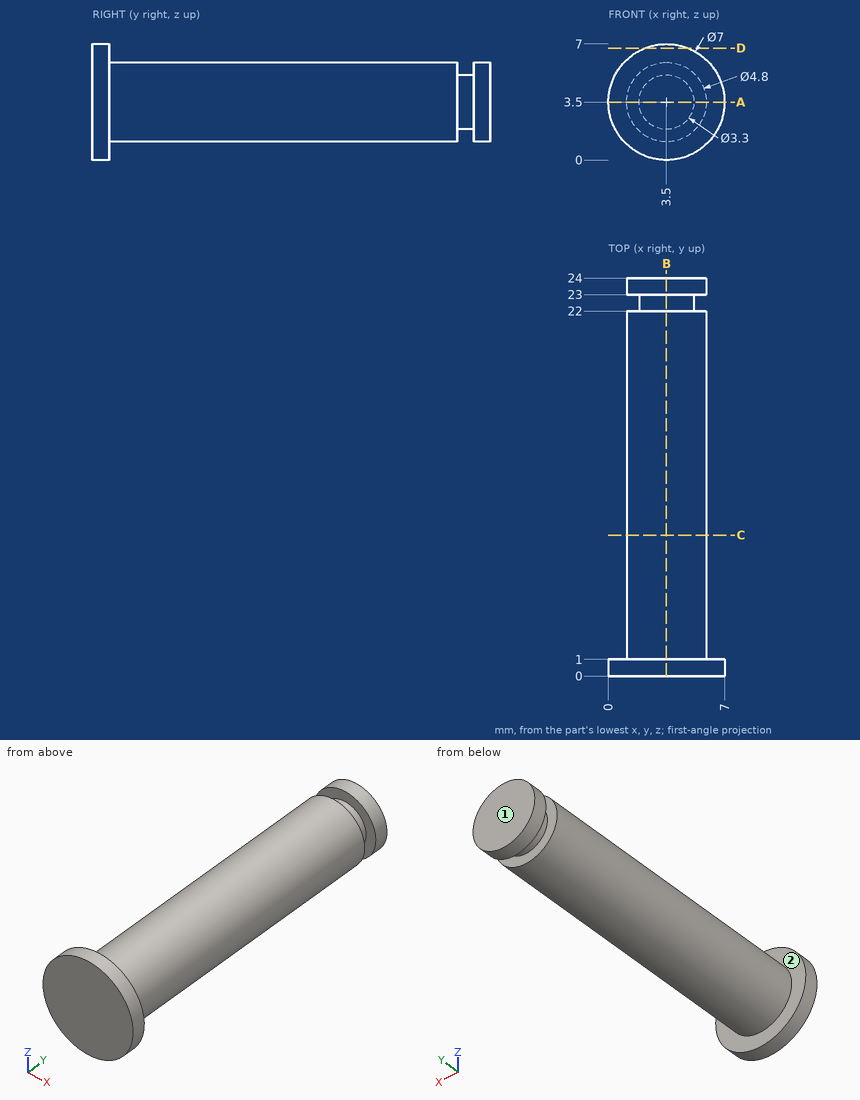
Here's the drawing with two shaded views (mm, measured from the low corner). I have some questions. A direction names the side the tool comes from. Give positions to 0.01 mm unless a question says otherwise; leave off trailing zeros. Loops run counter-clockwise (first coordinate to the right, second up) from the corner with the lowest first, then second, coordinate; pieces in that order, holes last. Notation, with made-up numbers: M -6,36.25 L 25,36.25 A15 cw 25,61.25 Z; hole C 56.5,15 d2. An arc over 180 degrees is marked long. Use one line per item in the form item = value. Start each with the question number.
(1) On a 3-axis mill with a long thin cutter (end or side, diameter ignored), from which of +Z, -Z, +X, -X, +Y, -Y can I reach the whole of each face in a straight line? I mean the marked faces 1 and 2. Say none if no direction works.
(2) I'm going to push flat-ended pins straight in: P1, Ø3, axis at y = 11.5, z = 5.5, coming from the +X side; P2, Ø4, axis at x = 3, y = 7.5, coming from the +Z side; P3, Ø2, axis at y = 19.5, z = 1, coming from the -X side. Where does each tip first touch, or does it pass through?
(3) I want a section at C-C, the plane y = 8.5. Write out the boundary of the cut face in (x, z), and give its area (3 significant figures).
(4) I want a section at B-B, the plane x = 3.5. Write out the boundary of the cut face in (y, z).
(5) I want a section at D-D, the plane z = 6.75. Write out the boundary of the cut face in (x, y), and give its area (3 significant figures).
(6) I want a section at A-A, the plane z = 3.5. Write out the boundary of the cut face in (x, y).
(7) Please list where these lines run through material, in increasing order: line 1 (Y direction, x = 2, z = 4.25); line 2 (Y direction, x = 1.75, z = 1.5); line 3 (X direction, y = 13, z = 2.75).
Worked out:
q1.face_1 = +Z, -Z, +X, -X, +Y
q1.face_2 = +Y
q2.P1 = 5.85
q2.P2 = 5.9
q2.P3 = 1.63
q3.outline = C 3.5,3.5 d4.8
q3.area = 18.1 mm²
q4.outline = M 0,0 L 1,0 L 1,1.1 L 22,1.1 L 22,1.85 L 23,1.85 L 23,1.1 L 24,1.1 L 24,5.9 L 23,5.9 L 23,5.15 L 22,5.15 L 22,5.9 L 1,5.9 L 1,7 L 0,7 Z
q5.outline = M 2.2,0 L 4.8,0 L 4.8,1 L 2.2,1 Z
q5.area = 2.60 mm²
q6.outline = M 0,0 L 7,0 L 7,1 L 5.9,1 L 5.9,22 L 5.15,22 L 5.15,23 L 5.9,23 L 5.9,24 L 1.1,24 L 1.1,23 L 1.85,23 L 1.85,22 L 1.1,22 L 1.1,1 L 0,1 Z
q7.line_1 = 0 to 22, 23 to 24
q7.line_2 = 0 to 1
q7.line_3 = 1.22 to 5.78
